from build123d import *

# Parameters (mm, degrees)
BOSS_EXTRUDE2_DEPTH = 20
FILLET10_R          = 3
SKETCH2_R           = 6
CUT_EXTRUDE1_DEPTH  = 152.327459504
SKETCH3_R           = 25
BOSS_EXTRUDE6_DEPTH = 40
SKETCH5_R           = 17.5
BOSS_EXTRUDE7_DEPTH = 15
SKETCH6_R           = 10
CUT_EXTRUDE2_DEPTH  = 191.91883092
CHAMFER1_SIZE       = 1


with BuildPart() as part:
    # Sketch1 → Boss-Extrude2 (new, symmetric)
    with BuildSketch(Plane(origin=(0, 0, 0), x_dir=(1, 0, 0), z_dir=(0, 1, 0))):
        Polygon((0, 0), (0, 45), (20, 45), (20, 85), (50, 85), (50, 45), (70, 45), (70, 0), (80, 0), (80, 55), (60, 55), (60, 120), (10, 120), (10, 55), (-10, 55), (-10, 0), align=None)
    extrude(amount=BOSS_EXTRUDE2_DEPTH, both=True)

    # Fillet10
    fillet10_edges = [part.edges().sort_by_distance(p)[0] for p in [
        (-10, 0, 0),
        (80, 0, 0),
        (70, 0, 0),
        (0, 0, 0),
    ]]
    fillet(fillet10_edges, radius=FILLET10_R)

    # Sketch2 → Cut-Extrude1 (cut, through all)
    with BuildSketch(Plane(origin=(80, 0, 0), x_dir=(0, 0, -1), z_dir=(1, 0, 0))):
        with Locations((20, 0)):
            Circle(SKETCH2_R)
    extrude(amount=-CUT_EXTRUDE1_DEPTH, mode=Mode.SUBTRACT)

    # Sketch3 → Boss-Extrude6 (add, symmetric)
    with BuildSketch(Plane(origin=(0, 0, 0), x_dir=(1, 0, 0), z_dir=(0, 1, 0))):
        with Locations(Location((35, 120, 0), (0, 0, 270))):
            Circle(SKETCH3_R)
    extrude(amount=BOSS_EXTRUDE6_DEPTH, both=True)

    # Sketch5 → Boss-Extrude7 (add, symmetric)
    with BuildSketch(Plane(origin=(0, 40, 0), x_dir=(1, 0, 0), z_dir=(0, 1, 0))):
        with Locations(Location((35, 120, 0), (0, 0, 270))):
            Circle(SKETCH5_R)
    extrude(amount=BOSS_EXTRUDE7_DEPTH, both=True)

    # Sketch6 → Cut-Extrude2 (cut, through all)
    with BuildSketch(Plane(origin=(0, 55, 0), x_dir=(1, 0, 0), z_dir=(0, 1, 0))):
        with Locations(Location((35, 120, 0), (0, 0, 270))):
            Circle(SKETCH6_R)
    extrude(amount=-CUT_EXTRUDE2_DEPTH, mode=Mode.SUBTRACT)

    # Chamfer1
    chamfer1_edges = [part.edges().sort_by_distance(p)[0] for p in [
        (-10, 0, -14),
        (0, 0, -14),
        (70, 0, -14),
        (80, 0, -14),
    ]]
    chamfer(chamfer1_edges, length=CHAMFER1_SIZE)


solid = part.part
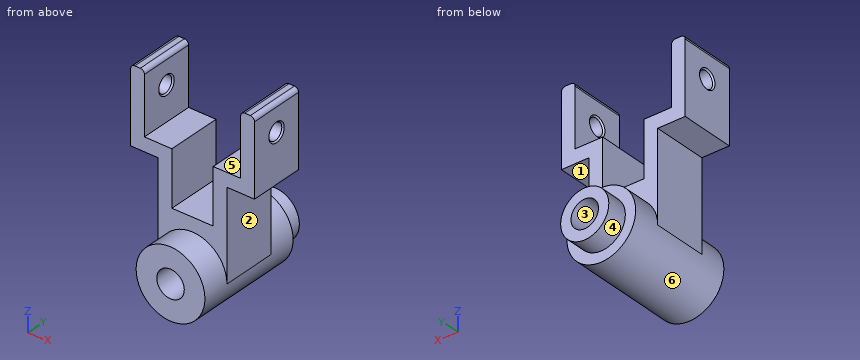
CAD build for the part. Positions are in the model's coordinates, mm. Face numbers are marked on the shaded views. A direction names the side the tool comes from. Round coordinates to 2 decimals unless told otherwise and drop trailing zeros. Write each loop counter-clockwise with the first axis right and the second up, starting at its lowest first coordinate (ties: lowest second). Pieces come first, ordered by that corner, then holes. Notation, with made-up numbers: M 71,-2 L 77,-2 A13 ccw 77,6 Z; hole C -8,-29 d11. An arc over 180 degrees is marked long. Use a Markdown table: item, result. Add a question column.
1. Pull direction X, two halves, no side cores. Call the marked faces 1, 2 and 3: released by +X, released by -X, zero draft, split by the parting line, or undercut.
2. Slice it at C-C on z = -65. Give the cut face in (x, y), then the cut area to 3 significant figures.
3. Flat gauge pins, fed straight in: P1, Ø10, axis at x = 68, y = 1.5, coming from the -Z side; P2, Ø15, axis at x = 32.5, y = 9, coming from the +Z side; P3, Ø3, axis at x = 58, y = 8, coming from the +Z side. Where does each tip first touch, or does it go through?
4. 3-axis set-ups, long thin cutter, end or side, ignore diameter. For the marked faces 4, 5 and 6: which of +Z, -Z, +X, -X, +Y, -Y reach the whole face in a straight line?
5. Slice it at D-D on y = 10.5. Give the cut face in (x, z), then the cut area to 3 significant figures.
6. Slice it at B-B on x = 35. Give the cut face in (y, z), then the cut area to 4 significant figures.
7. Drill centre lines: probe 1 along X at (y, z) = (15, -18); probe 2 along X at (y, z) = (17, -65); probe 3 along Y at (x, z) = (-3.5, -20). Where is each one in solid material? Low to high.
8. Slice it at A-A on z = -20. Give the cut face in (x, y), then the cut area to 3 significant figures.
Reply:
| question | item | result |
|---|---|---|
| 1 | face 1 | zero draft |
| 1 | face 2 | released by +X |
| 1 | face 3 | undercut |
| 2 | outline | M 10,-20 L 20,-20 L 20,20 L 10,20 Z; M 50,-20 L 60,-20 L 60,20 L 50,20 Z |
| 2 | area | 800 mm^2 |
| 3 | P1 | stops at z = -55 |
| 3 | P2 | stops at z = -85 |
| 3 | P3 | stops at z = -45 |
| 4 | face 4 | +Y |
| 4 | face 5 | +Z, +Y, -Y |
| 4 | face 6 | none |
| 5 | outline | M -10,-55 L 10,-55 L 10,-120 A25 ccw 60,-120 L 60,-55 L 80,-55 L 80,-3 A3 ccw 77,0 L 73,0 A3 ccw 70,-3 L 70,-45 L 50,-45 L 50,-85 L 20,-85 L 20,-45 L 0,-45 L 0,-3 A3 ccw -3,0 L -7,0 A3 ccw -10,-3 Z; hole C 35,-120 d20 |
| 5 | area | 4,510 mm^2 |
| 6 | outline | M -40,-145 L 40,-145 L 40,-137.5 L 55,-137.5 L 55,-130 L -40,-130 Z; M -40,-110 L 55,-110 L 55,-102.5 L 40,-102.5 L 40,-95 L 20,-95 L 20,-85 L -20,-85 L -20,-95 L -40,-95 Z |
| 6 | area | 3,025 mm^2 |
| 7 | probe 1 | x = -10 to 0, 70 to 80 |
| 7 | probe 2 | x = 10 to 20, 50 to 60 |
| 7 | probe 3 | y = -20 to -6, 6 to 20 |
| 8 | outline | M -10,-20 L 0,-20 L 0,-7 L -1,-6 L -9,-6 L -10,-7 Z; M -10,7 L -9,6 L -1,6 L 0,7 L 0,20 L -10,20 Z; M 70,-20 L 80,-20 L 80,-7 L 79,-6 L 71,-6 L 70,-7 Z; M 70,7 L 71,6 L 79,6 L 80,7 L 80,20 L 70,20 Z |
| 8 | area | 556 mm^2 |
